Could you check a few things on this drawing? It's one solid part, dimensions in mm from its lowest x, y, z. Coordinates: 2 decimals unless noted, no trailing zeros. Write each loop counter-clockwise with the first axis right and the second up, starting at its lowest first coordinate (ties: lowest second). Pieces come first, ordered by that corner, then holes. Notation, with made-up numbers: (-9.75, -3.75) - (45.25, -3.75) arc R14 cw to (45.25, 6.25) - close; hole circle Ø1 at (64, 86). An arc over 180 degrees is marked (long way). Answer as a JSON object with one key per item and string values. Group by question number.
1) If we section it at C-C (z = 8.75): State how many separate pieces and enclosed holes the cut face has, plus the area to 3 significant figures.
2) If we section it at A-A (x = 110): Write out the boundary of the cut face in (y, z).
3) Will these pins go through, and if not, where does the flat tip stop? pin 1 Ø10.5 at (x, y) = (70, 221) entering from +Z; pin 2 Ø8 at (x, y) = (89.5, 208.5) entering from -Z; pin 3 Ø1 at (x, z) = (153.5, 7) entering from +Y; pin 4 Ø3 at (y, z) = (132.5, 4.5) entering from +X.
4) If we section it at D-D (y = 246): Write out the boundary of the cut face in (x, z), plus the area to 3 significant figures.
5) If we section it at B-B (y = 126): Write out the boundary of the cut face in (x, z).
6) Please list where these lines run through material, in increasing order: line 1 along X through (y, z) = (234.5, 7.75) (1 decimal); line 2 along Y through (x, z) = (65, 7) (1 decimal); line 3 along Y through (x, z) = (163, 9.75) (1 decimal).
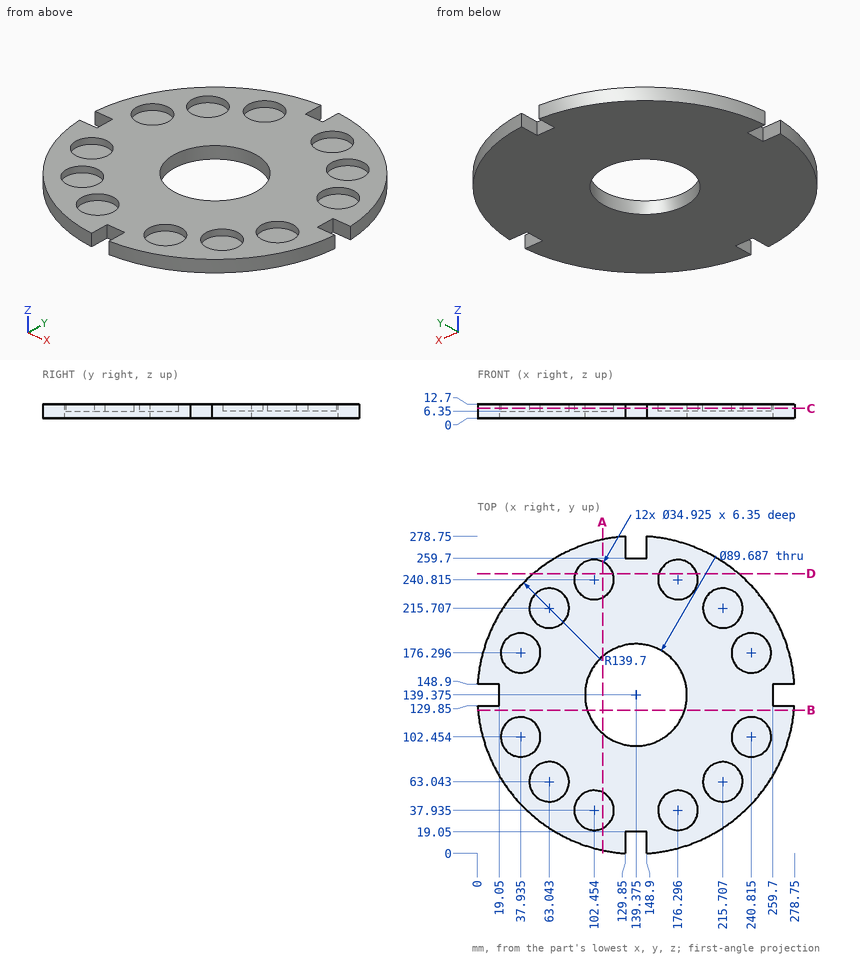
Here are the results:
{
 "1": {"separate pieces": "1", "enclosed holes": "13", "area": "42,000 mm²"},
 "2": {"outline": "(2.8, 0) - (105.49, 0) - (105.49, 12.7) - (53.68, 12.7) - (53.68, 6.35) - (22.19, 6.35) - (22.19, 12.7) - (2.8, 12.7) - close; (173.26, 0) - (275.95, 0) - (275.95, 12.7) - (256.56, 12.7) - (256.56, 6.35) - (225.07, 6.35) - (225.07, 12.7) - (173.26, 12.7) - close"},
 "3": {"pin 1": "stops at z = 6.35", "pin 2": "stops at z = 0", "pin 3": "stops at y = 278.41", "pin 4": "stops at x = 259.7"},
 "4": {"outline": "(49.11, 0) - (229.64, 0) - (229.64, 12.7) - (192.97, 12.7) - (192.97, 6.35) - (159.62, 6.35) - (159.62, 12.7) - (119.13, 12.7) - (119.13, 6.35) - (85.78, 6.35) - (85.78, 12.7) - (49.11, 12.7) - close", "area": "1,870 mm²"},
 "5": {"outline": "(0.32, 0) - (96.57, 0) - (96.57, 12.7) - (0.32, 12.7) - close; (182.18, 0) - (278.43, 0) - (278.43, 12.7) - (182.18, 12.7) - close"},
 "6": {"line 1": "x = 37.1 to 86.2, 118.7 to 160, 192.6 to 241.7", "line 2": "y = 21.1 to 45.7, 80.4 to 198.4, 233.1 to 257.6", "line 3": "y = 1.7 to 26.6, 49.3 to 101.3, 177.5 to 229.5, 252.1 to 277.1"}
}
